```python
from build123d import *

# Parameters (mm, degrees)
BASE_DEPTH                                 = 5.9944
WHEEL_CUTOUT_REACH                         = 145.809
SKETCH3_W                                  = 69.85
SKETCH3_H                                  = 25.4
WHEEL_CUTOUT_FILLETS_R                     = 3.175
WHEEL_CUTOUT_PATTERN_COUNT                 = 4
WHEEL_CUTOUT_FILLETS_OF_WHEEL_CUTOUT_PAT_R = 3.175
OUTSIDE_FILLETS_R                          = 6.35
F_8_CLEARANCE_HOLE1_D                      = 4.4958
CIRPATTERN2_COUNT                          = 4


with BuildPart() as part:
    # Base sketch → Base (new body)
    with BuildSketch(Plane(origin=(0, 0, 0), x_dir=(1, 0, 0), z_dir=(0, 1, 0))):
        Polygon((-101.6, 42.084097937), (-101.6, -42.084097937), (-42.084097937, -101.6), (42.084097937, -101.6), (101.6, -42.084097937), (101.6, 42.084097937), (42.084097937, 101.6), (-42.084097937, 101.6), align=None)
    extrude(amount=BASE_DEPTH)

    # Sketch3 → Wheel cutout (cut, up to next)
    with BuildSketch(Plane(origin=(0, 5.9944, 0), x_dir=(1, 0, 0), z_dir=(0, 1, 0)), mode=Mode.PRIVATE) as wheel_cutout_sk1:
        with Locations((0, 76.2)):
            Rectangle(SKETCH3_W, SKETCH3_H)
    wheel_cutout_tool1 = extrude(wheel_cutout_sk1.sketch, amount=-WHEEL_CUTOUT_REACH, mode=Mode.PRIVATE) & part.part
    wheel_cutout = wheel_cutout_tool1.solids().sort_by_distance((0, 5.9944, -76.2))[0]
    add(wheel_cutout, mode=Mode.SUBTRACT)

    # Wheel cutout fillets
    wheel_cutout_fillets_edges = [part.edges().sort_by_distance(p)[0] for p in [
        (-34.925, 2.9972, -63.5),
        (-34.925, 2.9972, -88.9),
        (34.925, 2.9972, -88.9),
        (34.925, 2.9972, -63.5),
    ]]
    fillet(wheel_cutout_fillets_edges, radius=WHEEL_CUTOUT_FILLETS_R)

    # Wheel cutout pattern: Wheel cutout ×4 about axis
    wheel_cutout_pattern_axis = Axis((0, 0, 0), (0, 1, 0))
    for i in range(1, WHEEL_CUTOUT_PATTERN_COUNT):
        add(wheel_cutout.rotate(wheel_cutout_pattern_axis, i * 360 / WHEEL_CUTOUT_PATTERN_COUNT), mode=Mode.SUBTRACT)

    # Wheel cutout fillets of Wheel cutout pat
    wheel_cutout_fillets_of_wheel_cutout_pat_edges = [part.edges().sort_by_distance(p)[0] for p in [
        (-63.5, 2.9972, 34.925),
        (-88.9, 2.9972, 34.925),
        (-88.9, 2.9972, -34.925),
        (-63.5, 2.9972, -34.925),
        (34.925, 2.9972, 63.5),
        (34.925, 2.9972, 88.9),
        (-34.925, 2.9972, 88.9),
        (-34.925, 2.9972, 63.5),
        (63.5, 2.9972, -34.925),
        (88.9, 2.9972, -34.925),
        (88.9, 2.9972, 34.925),
        (63.5, 2.9972, 34.925),
    ]]
    fillet(wheel_cutout_fillets_of_wheel_cutout_pat_edges, radius=WHEEL_CUTOUT_FILLETS_OF_WHEEL_CUTOUT_PAT_R)

    # Outside fillets
    outside_fillets_edges = [part.edges().sort_by_distance(p)[0] for p in [
        (-42.084097937, 2.9972, -101.6),
        (42.084097937, 2.9972, -101.6),
        (101.6, 2.9972, -42.084097937),
        (101.6, 2.9972, 42.084097937),
        (42.084097937, 2.9972, 101.6),
        (-101.6, 2.9972, 42.084097937),
        (-101.6, 2.9972, -42.084097937),
    ]]
    fillet(outside_fillets_edges, radius=OUTSIDE_FILLETS_R)

    # #8 Clearance Hole1 (through all)
    with Locations(Plane(origin=(0, 5.9944, 0), x_dir=(1, 0, 0), z_dir=(0, 1, 0))):
        with Locations((0, 95.25), (-12.7, 95.25), (12.7, 95.25), (12.7, 57.15), (-12.7, 57.15), (0, 57.15)):
            f_8_clearance_hole1 = Hole(F_8_CLEARANCE_HOLE1_D / 2)

    # CirPattern2: #8 Clearance Hole1 ×4 about axis
    cirpattern2_axis = Axis((0, 0, 0), (0, 1, 0))
    for i in range(1, CIRPATTERN2_COUNT):
        add(f_8_clearance_hole1.rotate(cirpattern2_axis, i * 360 / CIRPATTERN2_COUNT), mode=Mode.SUBTRACT)


solid = part.part
```
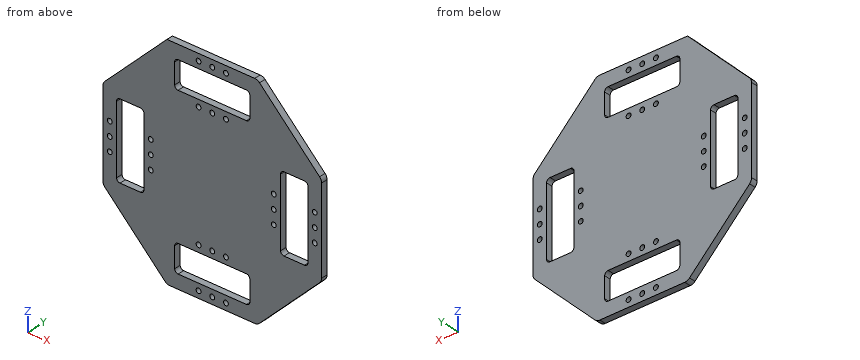
The listing builds one solid part. Answer for the finished solid, in the listing's coordinates (mm). Coordinates: 2 decimals unless noted, no trailing zeros. Write each loop counter-clockwise with the first axis right and the second up, starting at its lowest first coordinate (ties: lowest second). Pieces come first, ordered by that corner, then holes. Notation, with made-up numbers: M -2.5,43.5 L 21.5,43.5 A15 ccw 21.5,68.5 Z; hole C 31.5,38 d4. An arc over 180 degrees is marked long. Use a Markdown table: item, result. Add a question column.
1. Section B-B (y = 1.4) is taken. Count the separate pieces of the cut face and the enclosed holes in it, plus the area to 3 significant figures.
2. Section A-A (z = -82.5) is taken. Give the vertices of the cut face in (x, y) (3 decimals), plus the area to 3 significant figures.
3. Given P1, Ø3.5, axis at x = -12.7, z = 95.25, coming from the +Y side (3 decimals), flat-ended and moving along its own axis, determine where the tip first touches the part or whether it passes through.
4. Section C-C (z = 51.5) is taken. Give the vertices of the cut face in (x, y).
5. Straight lines are drawn through the part: line 1 along Z through (x, y) = (-4.5, 2.5); line 2 along Z through (x, y) = (77, 3.4) (3 decimals). For each, find the intervals that lie inside material, in ascending order. Write a range as [from, to].
Data:
| question | item | result |
|---|---|---|
| 1 | separate pieces | 1 |
| 1 | enclosed holes | 28 |
| 1 | area | 26,800 mm2 |
| 2 | outline | M -61.184,0 L -34.925,0 L -34.925,5.994 L -61.184,5.994 Z; M 34.925,0 L 61.184,0 L 61.184,5.994 L 34.925,5.994 Z |
| 2 | area | 315 mm2 |
| 3 | P1 | passes through |
| 4 | outline | M -92.18,0 L 92.18,0 L 92.18,5.99 L -92.18,5.99 Z |
| 5 | line 1 | z = [-101.6, -88.9], [-63.5, 63.5], [88.9, 101.6] |
| 5 | line 2 | z = [-66.684, -34.925], [34.925, 66.684] |
